Could you check a few things on this model? Use its own coordinates, in mm. Coordinates: 2 decimals unless noted, no trailing zeros. Order: outer loops, then holes, each group sorted by start corner. A loop starts at its lowest first (then second) coordinate and runs counter-clockwise, first axis right, second up. Notation, with made-up numbers: (67, 47) - (82, 47) arc R18 cw to (82, 73) - close; hole circle Ø7 at (-11, 60). An arc over 180 degrees is marked (long way). Answer as a JSON object with one key per item and string values. Group by question number.
(1) Imagine slicing it at C-C, the plane y = 4. Write out the boundary of the cut face in (x, z), and give its area (3 significant figures).
(2) Imagine slicing it at A-A, the plane z = 22. Write out the boundary of the cut face in (x, y), and give its area (3 significant figures).
(3) Please list where these lines run through material, in increasing order: probe 1 along Z at (x, y) = (16.75, -3.75); probe 2 along X at (y, z) = (2.75, 7); probe 3 along X at (y, z) = (-2.75, 19).
(4) Will these pins go through, and if not, where does the flat tip stop? P1, Ø1.5, axis at x = 24, z = 21, coming from the +Y side; P2, Ø1.5, axis at x = 24.5, z = 11.5, coming from the -Y side; P3, Ø1.5, axis at x = 10.5, z = 31, coming from the -Y side.
(5) Imagine slicing it at B-B, the plane x = 19.25. Write out the boundary of the cut face in (y, z).
from build123d import *

# Parameters (mm, degrees)
BOSS_EXTRUDE1_DEPTH = 40
CUT_EXTRUDE1_DEPTH  = 239


with BuildPart() as part:
    # Sketch1 → Boss-Extrude1 (new body)
    with BuildSketch(Plane.XY):
        with BuildLine():
            Line((30.047665389, 0), (30.047665389, 5.358567608))
            Line((30.047665389, 5.358567608), (1.215039634, -0.459096075))
            ThreePointArc((1.215039634, -0.459096075), (0.492690836, -0.825874412), (0.062707817, -1.512481095))
            Line((0.062707817, -1.512481095), (0.062707817, -1.945783899))
            ThreePointArc((0.062707817, -1.945783899), (0.484381365, -2.994370603), (1.514610899, -3.459096075))
            Line((1.514610899, -3.459096075), (30.047665389, -4.641432392))
            Line((30.047665389, -4.641432392), (30.047665389, 0))
        make_face()
    extrude(amount=BOSS_EXTRUDE1_DEPTH)

    # Sketch5 → Cut-Extrude1 (cut)
    with BuildSketch(Plane(origin=(-0.140494121, -3.390512784, 0), x_dir=(0.99914257391908, -0.04140189587876196, 0), z_dir=(-0.04140189587876195, -0.9991425739190799, 0))):
        with BuildLine():
            Line((16.27382087, 5.238645278), (16.27382087, 6.238645278))
            ThreePointArc((16.27382087, 6.238645278), (16.420267479, 6.592198669), (16.77382087, 6.738645278))
            Line((16.77382087, 6.738645278), (17.77382087, 6.738645278))
            Line((17.77382087, 6.738645278), (17.77382087, 7.738645278))
            Line((17.77382087, 7.738645278), (17.77382087, 8.738645278))
            Line((17.77382087, 8.738645278), (16.77382087, 8.738645278))
            ThreePointArc((16.77382087, 8.738645278), (16.420267479, 8.885091887), (16.27382087, 9.238645278))
            Line((16.27382087, 9.238645278), (16.27382087, 10.238645278))
            Line((16.27382087, 10.238645278), (14.27382087, 10.238645278))
            Line((14.27382087, 10.238645278), (14.27382087, 9.238645278))
            ThreePointArc((14.27382087, 9.238645278), (14.12737426, 8.885091887), (13.77382087, 8.738645278))
            Line((13.77382087, 8.738645278), (12.77382087, 8.738645278))
            Line((12.77382087, 8.738645278), (12.77382087, 6.738645278))
            Line((12.77382087, 6.738645278), (13.77382087, 6.738645278))
            ThreePointArc((13.77382087, 6.738645278), (14.12737426, 6.592198669), (14.27382087, 6.238645278))
            Line((14.27382087, 6.238645278), (14.27382087, 5.238645278))
            Line((14.27382087, 5.238645278), (15.27382087, 5.238645278))
            Line((15.27382087, 5.238645278), (16.27382087, 5.238645278))
        make_face()
    extrude(amount=-CUT_EXTRUDE1_DEPTH, mode=Mode.SUBTRACT)


solid = part.part
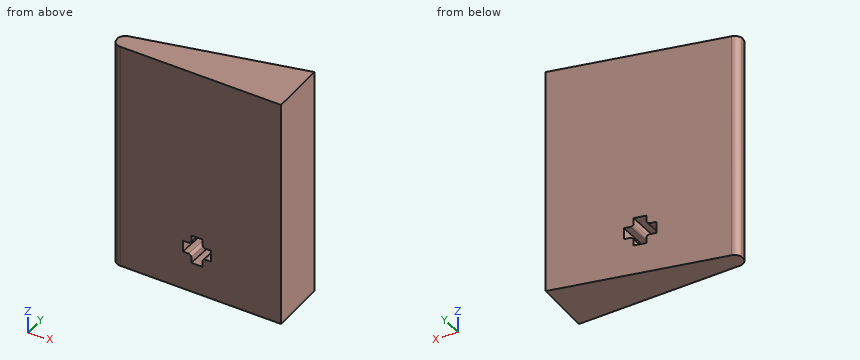
Result set:
{
 "1": {"outline": "(23.31, 0) - (30.05, 0) - (30.05, 40) - (23.31, 40) - close", "area": "269 mm^2"},
 "2": {"outline": "(0.06, -1.95) arc R1.51 ccw to (1.51, -3.46) - (30.05, -4.64) - (30.05, 5.36) - (1.22, -0.46) arc R1.51 ccw to (0.06, -1.51) - close", "area": "190 mm^2"},
 "3": {"probe 1": "z = 0 to 6.74, 8.74 to 40", "probe 2": "x = 17.9 to 30.05", "probe 3": "x = 0.29 to 30.05"},
 "4": {"P1": "stops at y = 4.29", "P2": "stops at y = -4.44", "P3": "stops at y = -3.86"},
 "5": {"outline": "(-4.19, 0) - (3.18, 0) - (3.18, 40) - (-4.19, 40) - close"}
}
